Could you check a few things on this model? Use its own coordinates, in mm. Face numbers are marked on the shaded views. A direction names the side the tool comes from. Give positions to 0.01 mm unless a question says otherwise; leave off trailing zeros. Write each loop counter-clockwise with the first axis right and the second up, starting at its lowest first coordinate (ties: lowest second). Pieces come first, ordered by that corner, then holes. Notation, with made-up numbers: M 63.5,7 L 86.5,7 A15 ccw 86.5,18 Z; hole C 34,-9 d1. An arc over 180 degrees is marked long. Answer as CSV lines item,"result". Start each with the question number.
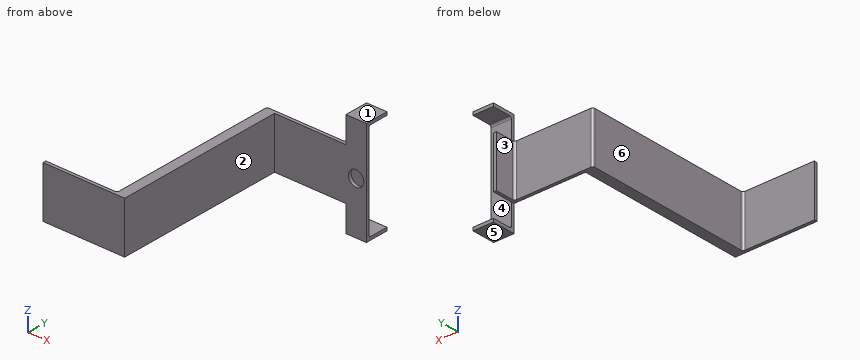
from build123d import *

# Parameters (mm, degrees)
SKETCH1_W           = 101.6
SKETCH1_H           = 63.5
BOSS_EXTRUDE1_DEPTH = 3.81
SKETCH2_W           = 12.7
SKETCH2_H           = 63.5
BOSS_EXTRUDE2_DEPTH = 212.09
SKETCH3_R           = 9.525
BOSS_EXTRUDE3_DEPTH = 3.81
SKETCH4_W           = 25.4
SKETCH4_H           = 3.841083916
SKETCH4_W_2         = 3.700866251
SKETCH4_H_2         = 63.5
SKETCH4_H_3         = 3.885733648
BOSS_EXTRUDE6_DEPTH = 25.4
SKETCH6_W           = 25.4
SKETCH6_H           = 3.885733648
SKETCH6_H_2         = 3.841083916
BOSS_EXTRUDE7_DEPTH = 3.81
FILLET2_R           = 2.54


with BuildPart() as part:
    # Sketch1 → Boss-Extrude1 (new body)
    with BuildSketch(Plane(origin=(0, 0, 0), x_dir=(1, 0, 0), z_dir=(0, 1, 0))):
        with Locations((50.8, -31.75)):
            Rectangle(SKETCH1_W, SKETCH1_H)
    extrude(amount=BOSS_EXTRUDE1_DEPTH)

    # Sketch2 → Boss-Extrude2 (add)
    with BuildSketch(Plane(origin=(0, 3.81, 0), x_dir=(1, 0, 0), z_dir=(0, 1, 0))):
        with Locations((95.25, -31.75)):
            Rectangle(SKETCH2_W, SKETCH2_H)
    extrude(amount=BOSS_EXTRUDE2_DEPTH)

    # Sketch3 → Boss-Extrude3 (add)
    with BuildSketch(Plane(origin=(0, 215.9, 0), x_dir=(1, 0, 0), z_dir=(0, 1, 0))):
        Polygon((101.6, 0), (190.5, 0), (190.5, 28.575), (203.2, 28.575), (215.9, 28.575), (215.9, -92.075), (203.2, -92.075), (190.5, -92.075), (190.5, -63.5), (101.6, -63.5), align=None)
        with Locations((203.2, -31.75)):
            Circle(SKETCH3_R, mode=Mode.SUBTRACT)
    extrude(amount=-BOSS_EXTRUDE3_DEPTH)

    # Sketch4 → Boss-Extrude6 (add)
    with BuildSketch(Plane(origin=(0, 215.9, 0), x_dir=(1, 0, 0), z_dir=(0, 1, 0))):
        with Locations((203.2, -93.995541958)):
            Rectangle(SKETCH4_W, SKETCH4_H)
        with Locations((188.649566875, -31.75)):
            Rectangle(SKETCH4_W_2, SKETCH4_H_2)
        with Locations((203.2, 30.517866824)):
            Rectangle(SKETCH4_W, SKETCH4_H_3)
    extrude(amount=BOSS_EXTRUDE6_DEPTH)

    # Sketch6 → Boss-Extrude7 (add)
    with BuildSketch(Plane.XZ.offset(-215.9)):
        with Locations((203.2, -30.517866824)):
            Rectangle(SKETCH6_W, SKETCH6_H)
        with Locations((203.2, 93.995541958)):
            Rectangle(SKETCH6_W, SKETCH6_H_2)
    extrude(amount=BOSS_EXTRUDE7_DEPTH)

    # Fillet2
    fillet2_edges = [part.edges().sort_by_distance(p)[0] for p in [
        (203.2, 215.9, -28.575),
        (88.9, 215.9, 31.75),
        (88.9, 3.81, 31.75),
        (186.799133749, 215.9, 31.75),
        (203.2, 215.9, 92.075),
    ]]
    fillet(fillet2_edges, radius=FILLET2_R)


solid = part.part
1. Please list where these lines run through material, in increasing order: line 1 (Z direction, x = 203.2, y = 214.45) (3 decimals); line 2 (X direction, y = 213, z = 31); line 3 (X direction, y = 215, z = 31).
2. Thinking about a two-plate mould opening in Z: for the marked faces 4, 5 and 6, which applies, pulls with the +Z half, pulls with the -Z half, needs draft (parallel to the pull), parting line crosses it, or undercut?
3. Imagine slicing it at D-D, the plane y = 87.5. Please give me the cut outline in (x, z).
4. Imagine slicing it at C-C, the plane z = 6. Please give me the cut outline in (x, y), plus the area to 3 significant figures.
5. Will these pins go through, and if not, where does the flat tip stop? P1, Ø25, axis at x = 203.2, z = 31.75, coming from the -Y side; P2, Ø18.5, axis at y = 230.5, z = 45, coming from the -X side; P3, Ø10, axis at x = 125.5, z = 29, coming from the +Y side; P4, Ø14.5, axis at y = 228.5, z = 77.5, coming from the -X side.
6. Imagine slicing it at B-B, the plane z = 31.75. Please give me the cut outline in (x, y) (3 decimals).
7. Imagine slicing it at A-A, the plane x = 203.2. Please give me the cut outline in (y, z) (3 decimals), plus the area to 3 significant figures.
8. On a 3-axis mill with a long thin cutter (end or side, diameter ignored), from which of +Z, -Z, +X, -X, +Y, -Y can I reach the whole of each face in a straight line? I mean the marked faces 1, 2 and 3. Say none if no direction works.
Solutions:
1,line 1,"-32.461 to 22.225, 41.275 to 95.916"
1,line 2,"88.9 to 193.7, 212.7 to 215.9"
1,line 3,"89.5 to 193.7, 212.7 to 215.9"
2,face 4,"undercut"
2,face 5,"pulls with the -Z half"
2,face 6,"needs draft"
3,outline,"M 88.9,0 L 101.6,0 L 101.6,63.5 L 88.9,63.5 Z"
4,outline,"M 0,0 L 101.6,0 L 101.6,212.09 L 215.9,212.09 L 215.9,215.9 L 190.5,215.9 L 190.5,241.3 L 186.8,241.3 L 186.8,218.44 A2.54 cw 184.26,215.9 L 91.44,215.9 A2.54 ccw 88.9,213.36 L 88.9,6.35 A2.54 cw 86.36,3.81 L 0,3.81 Z"
4,area,"3,610 mm²"
5,P1,"y = 212.09"
5,P2,"x = 186.8"
5,P3,"y = 215.9"
5,P4,"through"
6,outline,"M 0,0 L 101.6,0 L 101.6,212.09 L 193.675,212.09 L 193.675,215.9 L 190.5,215.9 L 190.5,241.3 L 186.799,241.3 L 186.799,218.44 A2.54 cw 184.259,215.9 L 91.44,215.9 A2.54 ccw 88.9,213.36 L 88.9,6.35 A2.54 cw 86.36,3.81 L 0,3.81 Z; M 212.725,212.09 L 215.9,212.09 L 215.9,215.9 L 212.725,215.9 Z"
7,outline,"M 212.09,-32.461 L 241.3,-32.461 L 241.3,-28.575 L 218.44,-28.575 A2.54 cw 215.9,-26.035 L 215.9,22.225 L 212.09,22.225 Z; M 212.09,41.275 L 215.9,41.275 L 215.9,89.535 A2.54 cw 218.44,92.075 L 241.3,92.075 L 241.3,95.916 L 212.09,95.916 Z"
7,area,"616 mm²"
8,face 1,"+Z, +X, -X, +Y, -Y"
8,face 2,"+Z, -Z, +X, -Y"
8,face 3,"+Z, -Z, -X, +Y"
